Part model, mm, in its own coordinate system. Give positions to 0.01 mm unless a question says otherwise; leave off trailing zeros. Write each loop counter-clockwise with the first axis right and the second up, starting at its lowest first coordinate (ties: lowest second). Pieces come first, ordered by that corner, then holes.
```python
from build123d import *

# Parameters (mm, degrees)
SKETCH1_W           = 500
SKETCH1_H           = 491
SKETCH1_R           = 110.5
SKETCH1_R_2         = 17.5
BOSS_EXTRUDE1_DEPTH = 10
CHAMFER1_SIZE       = 50


with BuildPart() as part:
    # Sketch1 → Boss-Extrude1 (new body)
    with BuildSketch(Plane(origin=(0, 0, 0), x_dir=(1, 0, 0), z_dir=(0, 1, 0))):
        Rectangle(SKETCH1_W, SKETCH1_H)
        with Locations((0, -35.5)):
            Circle(SKETCH1_R, mode=Mode.SUBTRACT)
        with Locations((-155, 124.5)):
            Circle(SKETCH1_R_2, mode=Mode.SUBTRACT)
        with Locations((155, 124.5)):
            Circle(SKETCH1_R_2, mode=Mode.SUBTRACT)
        with Locations((-155, -185.5)):
            Circle(SKETCH1_R_2, mode=Mode.SUBTRACT)
        with Locations((155, -185.5)):
            Circle(SKETCH1_R_2, mode=Mode.SUBTRACT)
    extrude(amount=BOSS_EXTRUDE1_DEPTH)

    # Chamfer1
    chamfer1_edges = [part.edges().sort_by_distance(p)[0] for p in [
        (250, 5, 245.5),
        (-250, 5, 245.5),
    ]]
    chamfer(chamfer1_edges, length=CHAMFER1_SIZE)


solid = part.part
```
1) Wall check: L1, parallel to Z at x = 155, y = 2.25; L2, parallel to X at y = 6.25, z = -124.5; L3, parallel to Z at x = 0, y = 5.5. Give the ranges that are in metal, low to high.
Answers follow:
L1: z = -245.5 to -142, -107 to 168, 203 to 245.5
L2: x = -250 to -172.5, -137.5 to 137.5, 172.5 to 250
L3: z = -245.5 to -75, 146 to 245.5
2) Saw through at A-A, the plane z = 35.5. Write the cut outline in (x, y), then the cut area to 3 significant figures.
Answers follow:
outline: (-250, 0) - (-110.5, 0) - (-110.5, 10) - (-250, 10) - close; (110.5, 0) - (250, 0) - (250, 10) - (110.5, 10) - close
area: 2,790 mm2
3) Saw through at C-C, the plane y = 3.25. Write the cut outline in (x, z).
Answers follow:
outline: (-250, -245.5) - (250, -245.5) - (250, 195.5) - (200, 245.5) - (-200, 245.5) - (-250, 195.5) - close; hole circle Ø35 at (-155, -124.5); hole circle Ø35 at (-155, 185.5); hole circle Ø221 at (0, 35.5); hole circle Ø35 at (155, -124.5); hole circle Ø35 at (155, 185.5)
4) Pin check, flat tip, straight feed: pin 1 Ø21 at (x, z) = (155, 185.5) entering from +Y. Stop position of the tip, or through.
Answers follow:
pin 1: passes through
5) Saw through at D-D, the plane z = -124.5. Write the cut outline in (x, y).
Answers follow:
outline: (-250, 0) - (-172.5, 0) - (-172.5, 10) - (-250, 10) - close; (-137.5, 0) - (137.5, 0) - (137.5, 10) - (-137.5, 10) - close; (172.5, 0) - (250, 0) - (250, 10) - (172.5, 10) - close
6) Saw through at B-B, the plane x = 0. Write the cut outline in (y, z).
Answers follow:
outline: (0, -245.5) - (10, -245.5) - (10, -75) - (0, -75) - close; (0, 146) - (10, 146) - (10, 245.5) - (0, 245.5) - close
7) Two-plate mould, pull along Z, no slides. Class faces 1 (the face through (142.102, 4.93, 173.673)), 2 (the face through (-3, 10, -113)), 3 (the face through (-157.28, 4.93, -141.85)), 4 (the face through (-224.65, 4.93, 220.85)): +Z half, -Z half, draft (parallel to the pull), parting line (faces both ways), or undercut.
Answers follow:
face 1: undercut
face 2: draft
face 3: undercut
face 4: +Z half
